Work out the finished part from the listing and answer in its coordinate system (mm). A direction names the side the tool comes from. Give positions to 0.01 mm unless a question says otherwise; leave off trailing zeros. Order: outer loops, then holes, each group sorted by start corner. A loop starts at its lowest first (then second) coordinate and runs counter-clockwise, first axis right, second up. Notation, with made-up numbers: (32.25, 80.5) - (59.25, 80.5) arc R33 cw to (59.25, 116.5) - close; hole circle Ø5 at (-22.5, -29). An arc over 180 degrees is marked (long way). Write each question's results on one line, items separated by ' | '.
from build123d import *

# Parameters (mm, degrees)
F1_DEPTH       = 2.5
F3_DEPTH       = 2.5
F4_W           = 50
F4_H           = 50
F5_DEPTH       = 5
F7_D           = 4
F7_CSINK_D     = 8
F7_CSINK_ANGLE = 90


with BuildPart() as f1:
    # F0 (on Front) → F1 (new body, symmetric)
    with BuildSketch(Plane.XZ):
        Polygon((-75, 3), (-75, 8), (-73, 8), (-73, 10), (-80, 10), (-80, -0.8), (-59, -5), (59, -5), (80, -0.8), (80, 10), (73, 10), (73, 8), (75, 8), (75, 3), (60, 0), (-60, 0), align=None)
    extrude(amount=F1_DEPTH, both=True)

    # F2 (on Right) → F3 (join, symmetric)
    with BuildSketch(Plane.YZ):
        Polygon((-135, 3), (-135, 8), (-133, 8), (-133, 10), (-140, 10), (-140, -0.8), (-119, -5), (119, -5), (140, -0.8), (140, 10), (133, 10), (133, 8), (135, 8), (135, 3), (120, 0), (-120, 0), align=None)
    extrude(amount=F3_DEPTH, both=True)

    # F4 (on Top) → F5 (join)
    with BuildSketch(Plane.XY):
        Rectangle(F4_W, F4_H)
    extrude(amount=-F5_DEPTH)

    # F7 (through all)
    with Locations(Plane.XY):
        with Locations((15, -15), (-15, -15), (-15, 15), (15, 15)):
            CounterSinkHole(F7_D / 2, F7_CSINK_D / 2, counter_sink_angle=F7_CSINK_ANGLE)


solid = f1.part
1. A tool of negligible diameter and unlimited length cuts with its end or side. For faces 1 (the face through (69, 0, -3)), 2 (the face through (-25, 14, -2)), 3 (the face through (-75, 0, 5)), 4 (the face through (2.5, -87, -2)), 5 (the face through (-14, -25, -2)), from which of +Z, -Z, +X, -X, +Y, -Y can it reach the whole face along a straight path? Write none if from no direction.
Answer list:
face 1: -Z, +X, +Y, -Y | face 2: +Z, -Z, -X, +Y | face 3: +Y, -Y | face 4: +Z, -Z, +X, -Y | face 5: +Z, -Z, -X, -Y
2. Determine the mould class of faces 6 (the face through (80, 0, 5)), 7 (the face through (0, 1, 0)), 8 (the face through (52, -2.5, -1)) for opening direction Y: +Y half, -Y half, draft (parallel to the pull), parting line (faces both ways), or undercut.
Answer list:
face 6: draft | face 7: undercut | face 8: -Y half
3. A cutting plane is placed at A-A, the plane y = -99. Write down the section's boundary in (x, z), then the cut area to 3 significant figures.
Answer list:
outline: (-2.5, -5) - (2.5, -5) - (2.5, 0) - (-2.5, 0) - close | area: 25.0 mm^2
4. Straight lines are drawn through the part: line 1 (X direction, y = -15, z = -2.55); line 2 (X direction, y = 14.5, z = -0.25). For each, find the intervals that lie inside material, in ascending order. Write a range as [from, to].
Answer list:
line 1: [-25, -17], [-13, 13], [17, 25] | line 2: [-25, -18.72], [-11.28, 11.28], [18.72, 25]
5. Given P1, Ø2.5, axis at y = 9.5, z = -1.5, coming from the -X side; P2, Ø7.5, axis at x = 40.5, z = -0.5, coming from the +Y side; P3, Ø7.5, axis at y = -87.5, z = 2.5, coming from the -X side; P4, Ø4.5, axis at x = -15, y = -15, coming from the -Z side, each flat-ended and moving along its own axis, determine where each tip first touches the part or whether it passes through.
Answer list:
P1: x = -25 | P2: y = 2.5 | P3: x = -2.5 | P4: z = -5
